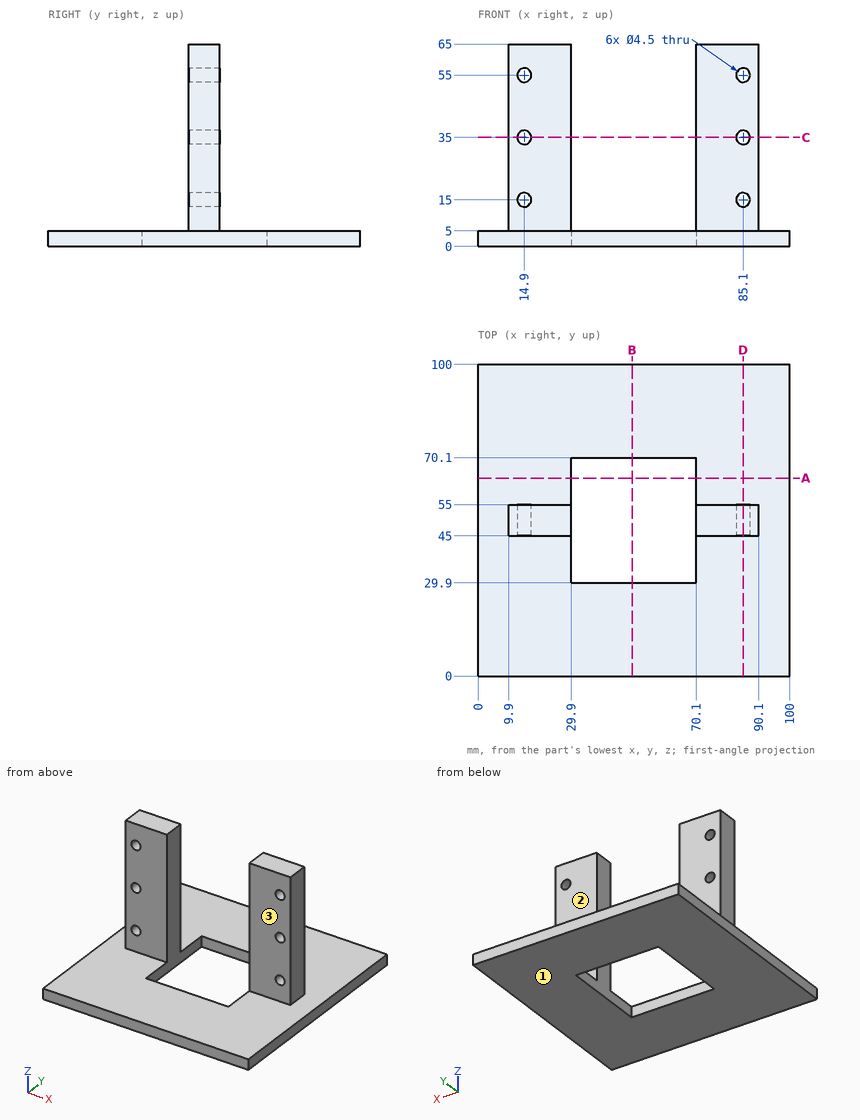
The drawing under review shows one solid part. Ordinate dimensions are in mm from its lowest x, y, z. A direction names the side the tool comes from. Coordinates: 2 decimals unless noted, no trailing zeros. Order: outer loops, then holes, each group sorted by start corner. A loop starts at its lowest first (then second) coordinate and runs counter-clockwise, first axis right, second up. Notation, with made-up numbers: (-11, 54) -> (23, 54) arc R23 ccw to (23, 89) -> close; hole circle Ø9 at (-29, 43). An arc over 180 degrees is marked (long way). Use CSV: the item, a comma, the result in double quotes. Start each with the question number.
Item 1: Wall thickness on probe 1 along Z at (x, y) = (14.9, 52.25); probe 2 along Z at (x, y) = (14, 49); probe 3 along Y at (x, z) = (17.5, 6.5): over which ranges is each line inside the solid? List them lowest first.
Item 2: Insertion check: pin 1 (5 mm diameter, centred on x = 85.1, z = 15, fed in from -Y); pin 2 (4 mm diameter, centred on x = 13.5, y = 80.5, fed in from +Z); pin 3 (8 mm diameter, centred on x = 74.5, z = 53.5, fed in from +Y); pin 4 (4 mm diameter, centred on x = 56, z = 1.5, fed in from -Y). Each pin has a flat end and moves straight along its axis. Give the tip position at first contact, or say it passes through.
Item 3: We need section D-D, the plane x = 85.1. Give the boundary of the cut face in (y, z).
Item 4: For the marked faces 1, 2 and 3, list the 3-axis set-ups (+Z, -Z, +X, -X, +Y, -Y) from which the entire face can be reached by the end or side of a thin tool; tool diameter is ignored.
Item 5: We need section A-A, the plane y = 63.5. Give the boundary of the cut face in (x, z).
Item 6: We need section C-C, the plane z = 35. Give the boundary of the cut face in (x, y).
Derived:
1,probe 1,"z = 0 to 12.75, 17.25 to 32.75, 37.25 to 52.75, 57.25 to 65"
1,probe 2,"z = 0 to 12.94, 17.06 to 32.94, 37.06 to 52.94, 57.06 to 65"
1,probe 3,"y = 45 to 55"
2,pin 1,"stops at y = 45"
2,pin 2,"stops at z = 5"
2,pin 3,"stops at y = 55"
2,pin 4,"stops at y = 0"
3,outline,"(0, 0) -> (100, 0) -> (100, 5) -> (55, 5) -> (55, 12.75) -> (45, 12.75) -> (45, 5) -> (0, 5) -> close; (45, 17.25) -> (55, 17.25) -> (55, 32.75) -> (45, 32.75) -> close; (45, 37.25) -> (55, 37.25) -> (55, 52.75) -> (45, 52.75) -> close; (45, 57.25) -> (55, 57.25) -> (55, 65) -> (45, 65) -> close"
4,face 1,"-Z, +X, -X, +Y, -Y"
4,face 2,"+Z, +X, -X, +Y"
4,face 3,"+Z, +X, -X, -Y"
5,outline,"(0, 0) -> (29.9, 0) -> (29.9, 5) -> (0, 5) -> close; (70.1, 0) -> (100, 0) -> (100, 5) -> (70.1, 5) -> close"
6,outline,"(9.9, 45) -> (12.65, 45) -> (12.65, 55) -> (9.9, 55) -> close; (17.15, 45) -> (29.9, 45) -> (29.9, 55) -> (17.15, 55) -> close; (70.1, 45) -> (82.85, 45) -> (82.85, 55) -> (70.1, 55) -> close; (87.35, 45) -> (90.1, 45) -> (90.1, 55) -> (87.35, 55) -> close"
